from build123d import *

# Parameters (mm, degrees)
PAD001_DEPTH      = 15
PAD001_DEPTH_BACK = 15
SKETCH014_W       = 12
SKETCH014_H       = 6
POCKET_DEPTH      = 28.001
SKETCH013_R       = 1.75
POCKET001_DEPTH   = 21
SKETCH012_R       = 5.15
POCKET002_DEPTH   = 43.001
SKETCH007_R       = 1.75
POCKET003_DEPTH   = 17.001
SKETCH008_W       = 6.407674
SKETCH008_H       = 16
SKETCH008_W_2     = 6.93002
SKETCH008_H_2     = 13.41794
POCKET004_DEPTH   = 31
SKETCH018_R       = 2
POCKET005_DEPTH   = 55.001
SKETCH020_W       = 2.261289
SKETCH020_H       = 2.342064
POCKET006_DEPTH   = 6
SKETCH015_W       = 50.47
SKETCH015_H       = 40
POCKET007_DEPTH   = 3
CHAMFER_SIZE      = 2
CHAMFER001_SIZE   = 2
CHAMFER002_SIZE   = 1
FILLET_R          = 3
FILLET001_R       = 1
FILLET002_R       = 1
FILLET003_R       = 1
FILLET004_R       = 1
FILLET005_R       = 1
FILLET006_R       = 1
FILLET007_R       = 1
FILLET008_R       = 1
FILLET009_R       = 1
FILLET010_R       = 1
FILLET011_R       = 1
FILLET012_R       = 1
FILLET013_R       = 1


with BuildPart() as part:
    # Sketch005 → Pad001 (new body, two sides)
    with BuildSketch(Plane.YZ) as pad001_sk:
        Polygon((0, -20), (0, 17), (3, 17), (3, 23), (-25, 23), (-25, 13), (-14, 13), (-14, -20), align=None)
    extrude(amount=PAD001_DEPTH)
    extrude(pad001_sk.sketch, amount=-PAD001_DEPTH_BACK)

    # Sketch014 (on Face5 of Pad001) → Pocket (cut, through all)
    with BuildSketch(Plane(origin=(0, -25, 0), x_dir=(0, 0, -1), z_dir=(0, -1, 0))):
        with Locations((-13, -5)):
            Rectangle(SKETCH014_W, SKETCH014_H)
    extrude(amount=-POCKET_DEPTH, mode=Mode.SUBTRACT)

    # Sketch013 → Pocket001 (cut)
    with BuildSketch(Plane(origin=(0, 0, 35), x_dir=(0, -1, 0), z_dir=(0, 0, 1))):
        with Locations((4, -5)):
            Circle(SKETCH013_R)
        with Locations((22, -5)):
            Circle(SKETCH013_R)
    extrude(amount=-POCKET001_DEPTH, mode=Mode.SUBTRACT)

    # Sketch012 (on Face4 of Pad001) → Pocket002 (cut, through all)
    with BuildSketch(Plane(origin=(0, 0, 23), x_dir=(0, -1, 0), z_dir=(0, 0, 1))):
        with Locations((13, -5)):
            Circle(SKETCH012_R)
    extrude(amount=-POCKET002_DEPTH, mode=Mode.SUBTRACT)

    # Sketch007 → Pocket003 (cut, through all)
    with BuildSketch(Plane(origin=(0, -14, 0), x_dir=(0, 0, -1), z_dir=(0, -1, 0))):
        with Locations((-6, 10)):
            Circle(SKETCH007_R)
        with Locations((14, 10)):
            Circle(SKETCH007_R)
        with Locations((-6, -10)):
            Circle(SKETCH007_R)
        with Locations((14, -10)):
            Circle(SKETCH007_R)
    extrude(amount=-POCKET003_DEPTH, mode=Mode.SUBTRACT)

    # Sketch008 → Pocket004 (cut)
    with BuildSketch(Plane.YX.offset(20)):
        with Locations((-11.703837, -8)):
            Rectangle(SKETCH008_W, SKETCH008_H)
        with Locations((-11.96501, 10.872729)):
            Rectangle(SKETCH008_W_2, SKETCH008_H_2)
    extrude(amount=-POCKET004_DEPTH, mode=Mode.SUBTRACT)

    # Sketch018 → Pocket005 (cut, through all)
    with BuildSketch(Plane(origin=(0, 0, 35), x_dir=(0, -1, 0), z_dir=(0, 0, 1))):
        with Locations((25.089622, 0)):
            Circle(SKETCH018_R)
    extrude(amount=-POCKET005_DEPTH, mode=Mode.SUBTRACT)

    # Sketch020 (on Face29 of Pocket005) → Pocket006 (cut)
    with BuildSketch(Plane.YX.offset(-13)):
        with Locations((-24.390742, -1.171032)):
            Rectangle(SKETCH020_W, SKETCH020_H)
    extrude(amount=-POCKET006_DEPTH, mode=Mode.SUBTRACT)

    # Sketch015 → Pocket007 (cut)
    with BuildSketch(Plane.ZX):
        with Locations((-9.235, 0)):
            Rectangle(SKETCH015_W, SKETCH015_H)
    extrude(amount=-POCKET007_DEPTH, mode=Mode.SUBTRACT)

    # Chamfer
    chamfer_edges = [part.edges().sort_by_distance(p)[0] for p in [
        (-8, -5.75, 7),
    ]]
    chamfer(chamfer_edges, length=CHAMFER_SIZE)

    # Chamfer001
    chamfer001_edges = [part.edges().sort_by_distance(p)[0] for p in [
        (-2, -5.75, 7),
    ]]
    chamfer(chamfer001_edges, length=CHAMFER001_SIZE)

    # Chamfer002
    chamfer002_edges = [part.edges().sort_by_distance(p)[0] for p in [
        (-3, -3, 8),
        (-5, -3, 7),
        (-7, -3, 8),
    ]]
    chamfer(chamfer002_edges, length=CHAMFER002_SIZE)

    # Fillet
    fillet_edges = [part.edges().sort_by_distance(p)[0] for p in [
        (-15, -25, 18),
        (15, -25, 18),
        (-15, 3, 20),
        (15, 3, 20),
    ]]
    fillet(fillet_edges, radius=FILLET_R)

    # Fillet001
    fillet001_edges = [part.edges().sort_by_distance(p)[0] for p in [
        (-15, -8.5, -4.5),
        (4.163759, -14, -4.5),
    ]]
    fillet(fillet001_edges, radius=FILLET001_R)

    # Fillet002
    fillet002_edges = [part.edges().sort_by_distance(p)[0] for p in [
        (0.05198, -14, -3.5),
    ]]
    fillet(fillet002_edges, radius=FILLET002_R)

    # Fillet003
    fillet003_edges = [part.edges().sort_by_distance(p)[0] for p in [
        (15, -14, 12),
        (15, -8.5, -4.5),
    ]]
    fillet(fillet003_edges, radius=FILLET003_R)

    # Fillet004
    fillet004_edges = [part.edges().sort_by_distance(p)[0] for p in [
        (-8, -25, 16),
    ]]
    fillet(fillet004_edges, radius=FILLET004_R)

    # Fillet005
    fillet005_edges = [part.edges().sort_by_distance(p)[0] for p in [
        (-15, -14, 12),
    ]]
    fillet(fillet005_edges, radius=FILLET005_R)

    # Fillet006
    fillet006_edges = [part.edges().sort_by_distance(p)[0] for p in [
        (0, -8.5, -4.5),
    ]]
    fillet(fillet006_edges, radius=FILLET006_R)

    # Fillet007
    fillet007_edges = [part.edges().sort_by_distance(p)[0] for p in [
        (4.163759, -8.5, -4.5),
    ]]
    fillet(fillet007_edges, radius=FILLET007_R)

    # Fillet008
    fillet008_edges = [part.edges().sort_by_distance(p)[0] for p in [
        (-15, -3, -2),
        (15, -3, -2),
    ]]
    fillet(fillet008_edges, radius=FILLET008_R)

    # Fillet009
    fillet009_edges = [part.edges().sort_by_distance(p)[0] for p in [
        (-8, 3, 18),
        (-2, 3, 18),
    ]]
    fillet(fillet009_edges, radius=FILLET009_R)

    # Fillet010
    fillet010_edges = [part.edges().sort_by_distance(p)[0] for p in [
        (-2, 0, 16.5),
        (-8, 0, 16.5),
    ]]
    fillet(fillet010_edges, radius=FILLET010_R)

    # Fillet011
    fillet011_edges = [part.edges().sort_by_distance(p)[0] for p in [
        (-15, 0, 16.5),
    ]]
    fillet(fillet011_edges, radius=FILLET011_R)

    # Fillet012
    fillet012_edges = [part.edges().sort_by_distance(p)[0] for p in [
        (15, 0, 16.5),
    ]]
    fillet(fillet012_edges, radius=FILLET012_R)

    # Fillet013
    fillet013_edges = [part.edges().sort_by_distance(p)[0] for p in [
        (1.997991, -25, 18),
    ]]
    fillet(fillet013_edges, radius=FILLET013_R)


solid = part.part
Verification items for the finished model (mm, model axes). A direction names the side the tool comes from. Give positions to 0.01 mm unless a question says otherwise; leave off trailing zeros. Write each loop counter-clockwise with the first axis right and the second up, starting at its lowest first coordinate (ties: lowest second). Pieces come first, ordered by that corner, then holes.
(1) Access from +Z, -Z, +X, -X, +Y, -Y to the whole of each face (thin tool, end or side, straight path). Record for faces 4 (the face through (-2.814, -3.507, 7.489)), 5 (the face through (3.863, -13.715, -4.717)), 6 (the face through (-7, -6, 8)), 7 (the face through (0, -11, -5)).
(2) Cross-section at C-C (y = -15.5). Enter the section's corners in (x, z), plus the area to 3 significant figures.
(3) Gauge pin test, flat ends, axial feed: pin 1 (2 mm diameter, centred on x = -10, y = -18, fed in from -Z); pin 2 (4.5 mm diameter, centred on x = -10, y = 1, fed in from -Z); pin 3 (6.5 mm diameter, centred on x = 9.5, z = -10.5, fed in from -Y). Record the tip position at first contact, or that the pin passes through.
(4) Cross-section at A-A (z = 12.5). Enter the section's corners in (x, y), plus the area to 3 significant figures.
(5) Cross-section at B-B (z = -15). Enter the section's corners in (x, y).
(6) Material ranges on line 1 (X direction, y = -4.25, z = -14); line 2 (Z direction, x = -9, y = -6.5); line 3 (Z direction, x = 7.5, y = -17.25), recorded low to high.
(7) Mould release check, pull along Z, two halves, no side actions. Record for faces 1 (the face through (11.5, -5.8, -14.9)), 2 (the face through (7, -19, 13)), 3 (the face through (0, -3, -2)): +Z half, -Z half, draft (parallel to the pull), parting line (faces both ways), or undercut.
(8) Cross-section at D-D (x = -11). Enter the section's corners in (y, z), plus the area to 3 significant figures.
Worked out:
1. face 4: +Y
1. face 5: -Z, +X, -Y
1. face 6: +Y, -Y
1. face 7: -Z, -X, -Y
2. outline: (-15, 13) - (-9.5, 13) - (-9.5, 23) - (-15, 23) - close; (-0.5, 13) - (15, 13) - (15, 23) - (-0.5, 23) - close
2. area: 210 mm2
3. pin 1: stops at z = 13
3. pin 2: stops at z = 16
3. pin 3: stops at y = -8.5
4. outline: (-15, -13) arc R1 ccw to (-14, -14) - (-10.05, -14) arc R5.15 cw to (-8, -8.81) - (-8, -3) - (-14, -3) arc R1 ccw to (-15, -4) - close; (-2, -8.81) arc R5.15 cw to (0.15, -13) arc R1 ccw to (1.15, -14) - (14, -14) arc R1 ccw to (15, -13) - (15, -4) arc R1 ccw to (14, -3) - (-2, -3) - close
4. area: 246 mm2
5. outline: (-15, -7.5) arc R1 ccw to (-14, -8.5) - (-11.44, -8.5) - (-11.44, -3) - (-14, -3) arc R1 ccw to (-15, -4) - close; (-8.56, -8.5) - (-7.5, -8.5) arc R5.15 cw to (-2.5, -8.5) - (-1, -8.5) arc R1 cw to (0, -9.5) - (0, -11.77) arc R5.15 cw to (0.15, -13) arc R1 ccw to (1.15, -14) - (3.16, -14) arc R1 ccw to (4.16, -13) - (4.16, -9.5) arc R1 cw to (5.16, -8.5) - (8.56, -8.5) - (8.56, -3) - (-8.56, -3) - close; (11.44, -8.5) - (14, -8.5) arc R1 ccw to (15, -7.5) - (15, -4) arc R1 ccw to (14, -3) - (11.44, -3) - close
6. line 1: x = -15 to -11.75, -8.25 to 8.25, 11.75 to 15
6. line 2: z = -20 to -15.44, -12.56 to 4.56, 7.44 to 23
6. line 3: z = 13 to 23
7. face 1: undercut
7. face 2: -Z half
7. face 3: draft
8. outline: (-25, 13) - (-14, 13) - (-14, 11) - (-8.5, 11) - (-8.5, 7.44) - (-3, 7.44) - (-3, 16) - (0, 16) - (0, 17) - (3, 17) - (3, 23) - (-25, 23) - close; (-8.5, -20) - (-3, -20) - (-3, -15.44) - (-8.5, -15.44) - close; (-8.5, -12.56) - (-3, -12.56) - (-3, 4.56) - (-8.5, 4.56) - close
8. area: 420 mm2
